Source: CAD feature listing. Evaluate the final solid. Frame: model axes, mm. Face numbers are marked on the shaded views. Coordinates: 2 decimals unless noted, no trailing zeros. Loops run counter-clockwise (first coordinate to the right, second up) from the corner with the lowest first, then second, coordinate; pieces in that order, holes last. Notation, with made-up numbers: (-4.75, 45) -> (5.25, 45) arc R24 ccw to (5.25, 65) -> close; hole circle Ø8 at (14, -23). An arc over 180 degrees is marked (long way). Answer as CSV lines item,"result".
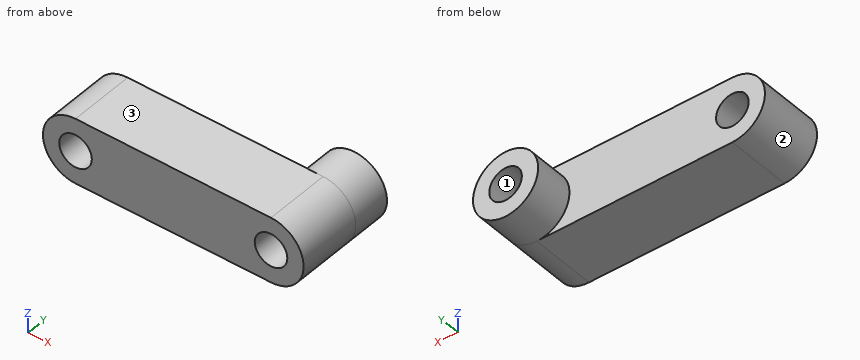
from build123d import *

# Parameters (mm, degrees)
BOSS_EXTRUDE1_DEPTH      = 4
BOSS_EXTRUDE1_DEPTH_BACK = 6
SKETCH1_R                = 2.5
BOSS_EXTRUDE3_DEPTH      = 11
BOSS_EXTRUDE3_DEPTH_BACK = 5
SKETCH3_R                = 5
SKETCH3_R_2              = 2.5


with BuildPart() as part:
    # Sketch1 → Boss-Extrude1 (new, two sides: drawn at the far end of the back side and taken through both)
    with BuildSketch(Plane(origin=(0, 0, 0), x_dir=(1, 0, 0), z_dir=(0, 1, 0)).offset(-BOSS_EXTRUDE1_DEPTH_BACK)):
        with BuildLine():
            Line((0, 5), (30, 5))
            ThreePointArc((30, 5), (35, 0), (30, -5))
            Line((30, -5), (0, -5))
            ThreePointArc((0, -5), (-5, 0), (0, 5))
        make_face()
        with Locations(Location((0, 0, 0), (0, 0, 270))):
            Circle(SKETCH1_R, mode=Mode.SUBTRACT)
        with Locations(Location((30, 0, 0), (0, 0, 270))):
            Circle(SKETCH1_R, mode=Mode.SUBTRACT)
    extrude(amount=BOSS_EXTRUDE1_DEPTH + BOSS_EXTRUDE1_DEPTH_BACK)

    # Sketch3 → Boss-Extrude3 (add, two sides: drawn at the far end of the back side and taken through both)
    with BuildSketch(Plane(origin=(0, -1, 0), x_dir=(1, 0, 0), z_dir=(0, 1, 0)).offset(-BOSS_EXTRUDE3_DEPTH_BACK)):
        with Locations(Location((30, 0, 0), (0, 0, 270))):
            Circle(SKETCH3_R)
        with Locations(Location((30, 0, 0), (0, 0, 270))):
            Circle(SKETCH3_R_2, mode=Mode.SUBTRACT)
    extrude(amount=BOSS_EXTRUDE3_DEPTH + BOSS_EXTRUDE3_DEPTH_BACK)


solid = part.part
(1) Draft query along X for the marked faces 1, 2 and 3. Return one class per face: released by +X, released by -X, zero draft, split by the parting line, or undercut.
Computed values:
face 1,"undercut"
face 2,"released by -X"
face 3,"zero draft"
(2) Cut plane B-B (y = -1.25). Return the cut outline in (x, z), then the cut area to 3 significant figures.
Computed values:
outline,"(0, -5) -> (30, -5) arc R5 ccw to (30, 5) -> (0, 5) arc R5 ccw to start; hole circle Ø5 at (0, 0); hole circle Ø5 at (30, 0)"
area,"339 mm^2"
(3) Pin query (flat end, axial travel): pin 1 Ø6 at (x, z) = (25.5, -2.5) entering from +Y; pin 2 Ø4 at (x, z) = (0, 0) entering from +Y; pin 3 Ø6 at (x, z) = (4, 3) entering from +Y. Return the tip coordinate at first contact, or that it passes through.
Computed values:
pin 1,"y = 10"
pin 2,"through"
pin 3,"y = 4"
(4) Cut plane C-C (x = 32). Return the cut outline in (y, z).
Computed values:
outline,"(-6, -4.58) -> (10, -4.58) -> (10, -1.5) -> (-6, -1.5) -> close; (-6, 1.5) -> (10, 1.5) -> (10, 4.58) -> (-6, 4.58) -> close"
(5) Cut plane D-D (x = 14.5). Return the cut outline in (y, z), then the cut area to 3 significant figures.
Computed values:
outline,"(-6, -5) -> (4, -5) -> (4, 5) -> (-6, 5) -> close"
area,"100 mm^2"
(6) Material intervals for L1, parallel to X at y = -1.25, z = 0; L2, parallel to X at y = -3.25, z = -2.25; L3, parallel to Y at x = 22, z = 2, sorted ascending. Write a range as [from, to].
Computed values:
L1,"[-5, -2.5], [2.5, 27.5], [32.5, 35]"
L2,"[-4.47, -1.09], [1.09, 28.91], [31.09, 34.47]"
L3,"[-6, 4]"
(7) Cut plane A-A (z = 0). Return the cut outline in (x, y).
Computed values:
outline,"(-5, -6) -> (-2.5, -6) -> (-2.5, 4) -> (-5, 4) -> close; (2.5, -6) -> (27.5, -6) -> (27.5, 10) -> (25, 10) -> (25, 4) -> (2.5, 4) -> close; (32.5, -6) -> (35, -6) -> (35, 10) -> (32.5, 10) -> close"
